The model under review builds one solid part; all positions refer to its coordinate system, in mm. Round coordinates to 2 decimals unless told otherwise and drop trailing zeros. Order: outer loops, then holes, each group sorted by start corner. A loop starts at its lowest first (then second) coordinate and runs counter-clockwise, first axis right, second up. Notation, with made-up numbers: (-21.5, 18.5) -> (-2.5, 18.5) arc R27 cw to (-2.5, 49.5) -> close; hole circle Ø3 at (16.5, 2). An arc over 180 degrees is marked (long way). Use a Markdown table: item, result. Add a question column.
```python
from build123d import *

# Parameters (mm, degrees)
SKETCH1_R           = 20
BOSS_EXTRUDE1_DEPTH = 200
BOSS_EXTRUDE1_TAPER = 1
SKETCH3_R           = 18
CUT_EXTRUDE1_DEPTH  = 200
CUT_EXTRUDE1_TAPER  = 1


with BuildPart() as part:
    # Sketch1 → Boss-Extrude1 (new body)
    with BuildSketch(Plane(origin=(0, 0, 0), x_dir=(1, 0, 0), z_dir=(0, 1, 0))):
        Circle(SKETCH1_R)
    extrude(amount=BOSS_EXTRUDE1_DEPTH, taper=BOSS_EXTRUDE1_TAPER)

    # Sketch3 → Cut-Extrude1 (cut)
    with BuildSketch(Plane.XZ):
        Circle(SKETCH3_R)
    extrude(amount=-CUT_EXTRUDE1_DEPTH, taper=CUT_EXTRUDE1_TAPER, mode=Mode.SUBTRACT)

    # Sketch4 → Revolve1 (revolve)
    with BuildSketch(Plane.XY):
        with BuildLine():
            Line((0, 227.660840397), (0, 225.660840397))
            add(Edge.make_bspline(
                [(0, 225.660840397), (3.662215859, 224.429250128), (11.624405947, 218.277965679), (14.357854187, 208.68709829), (14.508987014, 200)],
                knots=[0, 0, 0, 0, 0.332210555, 1, 1, 1, 1], degree=3))
            Line((14.508987014, 200), (16.508987014, 200))
            add(Edge.make_bspline(
                [(0, 227.660840397), (16.165150369, 220.569430353), (16.508987014, 200)],
                knots=[0, 0, 0, 1, 1, 1], degree=2))
        make_face()
    revolve(axis=Axis((0, 220.606902542, 0), (0, -1, 0)))


solid = part.part
```
Q1. Wall thickness on line 1 (Z direction, x = -3, y = 160.5); line 2 (X direction, y = 156.5, z = 12.5); line 3 (X direction, y = 172, z = 4): over which ranges is each line inside the solid? List them lowest first. Write a range as [from, to].
Q2. Add section A-A (y = 136). Write out the cut boundary in (x, z).
Q3. Add section B-B (y = 91.5). Write out the cut boundary in (x, z), then the cut area to 3 significant figures.
Q4. Mouldability with a two-part tool opening along X and no side actions: class faces 1 (the conical face through (-14.47, 101.4, 11.09)), 2 (the flat face through (-18, 0, -3)), 3 (the conical face through (15.48, 101.4, 4.88)) as pulls with the +X half, pulls with the -X half, needs draft (parallel to the pull), parting line crosses it, or undercut.
Q5. Insertion check: pin 1 (5 mm diameter, centred on y = 163.5, z = -7.5, fed in from -X); pin 2 (8 mm diameter, centred on x = 0.5, y = 145.5, fed in from +Z); pin 3 (3 mm diameter, centred on y = 119, z = -8, fed in from -X). Each pin has a flat end and moves straight along its axis. Give the tip position at first contact, or say it passes through.
Report:
| question | item | result |
|---|---|---|
| 1 | line 1 | z = [-16.93, -14.9], [14.9, 16.93] |
| 1 | line 2 | x = [-11.91, -8.77], [8.77, 11.91] |
| 1 | line 3 | x = [-16.52, -14.45], [14.45, 16.52] |
| 2 | outline | circle Ø35.25 at (0, 0); hole circle Ø31.25 at (0, 0) |
| 3 | outline | circle Ø36.81 at (0, 0); hole circle Ø32.81 at (0, 0) |
| 3 | area | 219 mm² |
| 4 | face 1 | parting line crosses it |
| 4 | face 2 | needs draft |
| 4 | face 3 | undercut |
| 5 | pin 1 | stops at x = -16.4 |
| 5 | pin 2 | stops at z = 17.53 |
| 5 | pin 3 | stops at x = -16.7 |
